```python
from build123d import *

# Parameters (mm, degrees)
F0_W     = 1.8
F0_H     = 10
F0_W_2   = 39.4
F0_H_2   = 7
F0_H_3   = 3
F1_DEPTH = 5
F2_DEPTH = 2
F3_START = -2.2
F3_DEPTH = 1.8
F4_START = -2
F4_DEPTH = 2
F5_DEPTH = 15
F6_R     = 5


with BuildPart() as f1:
    # F0 (on Top) → F1 (new body)
    with BuildSketch(Plane.XY):
        with Locations((-23.6, 0)):
            Rectangle(F0_W, F0_H)
        Polygon((-19.7, -2), (-19.7, 5), (-22.7, 5), (-22.7, -5), (-19.7, -5), align=None)
        with Locations((0, 1.5)):
            Rectangle(F0_W_2, F0_H_2)
        Polygon((22.7, -5), (22.7, 5), (19.7, 5), (19.7, -2), (19.7, -5), align=None)
        with Locations((23.6, 0)):
            Rectangle(F0_W, F0_H)
        with Locations((0, -3.5)):
            Rectangle(F0_W_2, F0_H_3)
    extrude(amount=F1_DEPTH)

    # F0 (on Top) → F2 (join)
    with BuildSketch(Plane.XY):
        with Locations((-23.6, 0)):
            Rectangle(F0_W, F0_H)
        with Locations((23.6, 0)):
            Rectangle(F0_W, F0_H)
    extrude(amount=-F2_DEPTH)



with BuildPart() as f3:
    # F0 (on Top) → F3 (new body)
    with BuildSketch(Plane.XY.offset(F3_START)):
        Polygon((-19.7, -2), (-19.7, 5), (-22.7, 5), (-22.7, -5), (-19.7, -5), align=None)
    extrude(amount=-F3_DEPTH)


with BuildPart() as f3b:
    # F0 (on Top) → F3, piece 2 (new body)
    with BuildSketch(Plane.XY.offset(F3_START)):
        Polygon((22.7, -5), (22.7, 5), (19.7, 5), (19.7, -2), (19.7, -5), align=None)
    extrude(amount=-F3_DEPTH)


with BuildPart() as f1_1:
    add(f1.part)

    add(f3.part)  # F4 merges F3

    add(f3b.part)  # F4 merges F3b
    # F0 (on Top) → F4 (join)
    with BuildSketch(Plane.XY.offset(F4_START)):
        with Locations((-23.6, 0)):
            Rectangle(F0_W, F0_H)
        with Locations((23.6, 0)):
            Rectangle(F0_W, F0_H)
    extrude(amount=-F4_DEPTH)

    # F0 (on Top) → F5 (join)
    with BuildSketch(Plane.XY):
        with Locations((0, -3.5)):
            Rectangle(F0_W_2, F0_H_3)
    extrude(amount=F5_DEPTH)

    # F6
    f6_edges = [f1_1.edges().sort_by_distance(p)[0] for p in [
        (-19.7, -3.5, 15),
        (19.7, -3.5, 15),
    ]]
    fillet(f6_edges, radius=F6_R)


solid = f1_1.part
```
Can you work these out from the model? Positions are in its coordinate system, mm. A direction names the side the tool comes from. Give positions to 0.01 mm unless a question says otherwise; leave off trailing zeros. Loops run counter-clockwise (first coordinate to the right, second up) from the corner with the lowest first, then second, coordinate; pieces in that order, holes last. Notation, with made-up numbers: M -32,51.5 L 6,51.5 A6 ccw 6,55.5 Z; hole C 36.25,-38 d9. An arc over 180 degrees is marked long. One line per question, with ' | ' between items. Start each with the question number.
Q1. For pin 1 Ø0.9 at (x, y) = (-21, 1) entering from +Z; pin 2 Ø8 at (x, z) = (-0.5, 11) entering from +Y; pin 3 Ø0.9 at (y, z) = (-3.5, 7.5) entering from +X, each with a flat end and sliding along its axis, tell me the tip position at first contact or that it passes through.
Q2. If we section it at A-A (z = -0.5): Please give me the cut outline in (x, y), plus the area to 3 significant figures.
Q3. If we section it at C-C (y = -2.75): Please give me the cut outline in (x, z).
Q4. If we mould it in two halves opening along Z, with no side actions, what happens to faces 1 (the flat face through (24.5, 0, 0)), 2 (the flat face through (-22.7, 0, -1)), 3 (the flat face through (22, 0, -4)), 4 (the cylindrical face through (18.2, -3.48, 13.57))? For each: +Z half, -Z half, draft (parallel to the pull), parting line (faces both ways), or undercut.
Q5. If we section it at B-B (x = -21): Please give me the cut outline in (y, z), plus the area to 3 significant figures.
Q6. If I drill on line 1 (Z direction, x = -21, y = 0.25); line 2 (Y direction, x = -14, z = 13.25); line 3 (X direction, y = -1.25, z = -1), over which ranges is the centre line in solid material (lowest first)? Write a range as from..to.
Q7. If we section it at D-D (x = 4.5): Please give me the cut outline in (y, z), plus the area to 3 significant figures.
Q8. For faces 5 (the flat face through (-19.7, -4, 7)), 6 (the flat face through (19.7, -4, 7)), 7 (the flat face through (0, 0, 0)), 8 (the flat face through (0, -2, 10)), which set-ups out of +Z, -Z, +X, -X, +Y, -Y let a thin tool reach every point of the face, with its end or its side?
Computed:
1) pin 1: stops at z = 5 | pin 2: stops at y = -2 | pin 3: stops at x = 19.7
2) outline: M -24.5,-5 L -22.7,-5 L -22.7,5 L -24.5,5 Z; M 22.7,-5 L 24.5,-5 L 24.5,5 L 22.7,5 Z | area: 36.0 mm²
3) outline: M -24.5,-4 L -19.7,-4 L -19.7,-2.2 L -22.7,-2.2 L -22.7,0 L 22.7,0 L 22.7,-2.2 L 19.7,-2.2 L 19.7,-4 L 24.5,-4 L 24.5,5 L 19.7,5 L 19.7,10 A5 ccw 14.7,15 L -14.7,15 A5 ccw -19.7,10 L -19.7,5 L -24.5,5 Z
4) face 1: draft | face 2: undercut | face 3: -Z half | face 4: +Z half
5) outline: M -5,-4 L 5,-4 L 5,-2.2 L -5,-2.2 Z; M -5,0 L 5,0 L 5,5 L -5,5 Z | area: 68.0 mm²
6) line 1: z = -4..-2.2, 0..5 | line 2: y = -5..-2 | line 3: x = -24.5..-22.7, 22.7..24.5
7) outline: M -5,0 L 5,0 L 5,5 L -2,5 L -2,15 L -5,15 Z | area: 80.0 mm²
8) face 5: +Z, -X, +Y, -Y | face 6: +Z, +X, +Y, -Y | face 7: +Y, -Y | face 8: +Z, +X, -X, +Y
